Check sheet for the modelled part. Datum: model origin and axes. Units: mm. Face numbers are marked on the shaded views. A direction names the side the tool comes from. Round coordinates to 2 decimals unless told otherwise and drop trailing zeros. Write each loop counter-clockwise with the first axis right and the second up, starting at its lowest first coordinate (ties: lowest second). Pieces come first, ordered by that corner, then holes. Notation, with made-up numbers: (9, 67) -> (13, 67) arc R7 cw to (13, 80) -> close; hole circle Ø7 at (54, 64.25). An arc over 180 degrees is marked (long way). Answer as a JSON object with one key per item and string values. Group by question number.
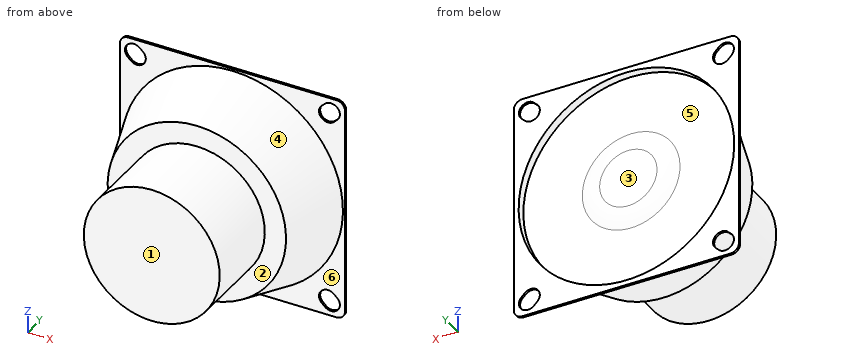
```python
from build123d import *

# Parameters (mm, degrees)
ESQUISSE2_R             = 16
BOSS_EXTRU_1_DEPTH      = 19
ESQUISSE3_R             = 21
BOSS_EXTRU_2_DEPTH      = 15
D_POUILLE1_ANGLE        = 18.5
BOSS_EXTRU_3_DEPTH      = 0.5
ESQUISSE5_R             = 25.375
ENL_V_MAT_EXTRU_1_DEPTH = 2
ESQUISSE6_R             = 11.5
BOSS_EXTRU_4_DEPTH      = 1.2
CONG_1_R                = 10
ENL_V_MAT_EXTRU_2_DEPTH = 10


with BuildPart() as part:
    # Esquisse2 → Boss.-Extru.1 (new body)
    with BuildSketch(Plane(origin=(0, 0, 0), x_dir=(1, 0, 0), z_dir=(0, 1, 0))):
        with Locations(Location((0, 0, 0), (0, 0, 270))):
            Circle(ESQUISSE2_R)
    extrude(amount=BOSS_EXTRU_1_DEPTH)

    # Esquisse3 → Boss.-Extru.2 (add)
    with BuildSketch(Plane(origin=(0, 19, 0), x_dir=(1, 0, 0), z_dir=(0, 1, 0))):
        with Locations(Location((0, 0, 0), (0, 0, 270))):
            Circle(ESQUISSE3_R)
    extrude(amount=BOSS_EXTRU_2_DEPTH)

    # Dépouille1
    d_pouille1_faces = [part.faces().sort_by_distance(p)[0] for p in [
        (0, 26.5, -21),
    ]]
    draft(d_pouille1_faces, Plane(origin=(0, 19, 0), x_dir=(0, 0, -1), z_dir=(0, -1, 0)), D_POUILLE1_ANGLE)

    # Esquisse4 → Boss.-Extru.3 (add)
    with BuildSketch(Plane(origin=(0, 34, 0), x_dir=(1, 0, 0), z_dir=(0, 1, 0))):
        with BuildLine():
            Line((-24.5, 26.5), (24.5, 26.5))
            ThreePointArc((24.5, 26.5), (25.914213562, 25.914213562), (26.5, 24.5))
            Line((26.5, 24.5), (26.5, -24.5))
            ThreePointArc((26.5, -24.5), (25.914213562, -25.914213562), (24.5, -26.5))
            Line((24.5, -26.5), (-24.5, -26.5))
            ThreePointArc((-24.5, -26.5), (-25.914213562, -25.914213562), (-26.5, -24.5))
            Line((-26.5, -24.5), (-26.5, 24.5))
            ThreePointArc((-26.5, 24.5), (-25.914213562, 25.914213562), (-24.5, 26.5))
        make_face()
    extrude(amount=BOSS_EXTRU_3_DEPTH)

    # Esquisse5 → Enlèv. mat.-Extru.1 (cut)
    with BuildSketch(Plane(origin=(0, 34.5, 0), x_dir=(1, 0, 0), z_dir=(0, 1, 0))):
        with Locations(Location((0, 0, 0), (0, 0, 270))):
            Circle(ESQUISSE5_R)
    extrude(amount=-ENL_V_MAT_EXTRU_1_DEPTH, mode=Mode.SUBTRACT)

    # Esquisse6 → Boss.-Extru.4 (add)
    with BuildSketch(Plane(origin=(0, 32.5, 0), x_dir=(1, 0, 0), z_dir=(0, 1, 0))):
        with Locations(Location((0, 0, 0), (0, 0, 270))):
            Circle(ESQUISSE6_R)
    extrude(amount=BOSS_EXTRU_4_DEPTH)

    # Congé1
    # the kernel refuses this fillet: 10 mm, written as the material it takes off along each edge
    with BuildSketch(Plane(origin=(0, 33.7, 0), x_dir=(0, 0, 1), z_dir=(-1, 0, 0))) as cong_1_piece_1:
        with BuildLine():
            CenterArc((6.750263165, -10), CONG_1_R, 61.642363424, 28.357636576)
            Line((6.750263165, 0), (6.750263165, 0.2))
            Line((6.750263165, 0.2), (11.5, 0.2))
            Line((11.5, 0.2), (11.7, 0))
            ThreePointArc((11.7, 0), (11.7, -0.6), (11.594994737, -1.024))
            Line((11.594994737, -1.024), (11.5, -1.2))
        make_face()
    revolve(axis=Axis((0, 33.7, 0), (0, 1, 0)), mode=Mode.SUBTRACT)

    # Esquisse7 → Enlèv. mat.-Extru.2 (cut)
    with BuildSketch(Plane(origin=(0, 34.5, 0), x_dir=(1, 0, 0), z_dir=(0, 1, 0))):
        with BuildLine():
            Line((21.024040871, 24.065615546), (21.74268552, 24.760993047))
            ThreePointArc((21.74268552, 24.760993047), (24.712132034, 24.712132034), (24.663271022, 21.74268552))
            Line((24.663271022, 21.74268552), (23.944626373, 21.04730802))
            ThreePointArc((23.944626373, 21.04730802), (20.975179858, 21.096169032), (21.024040871, 24.065615546))
        make_face()
        with BuildLine():
            Line((-21.024040871, 24.065615546), (-21.74268552, 24.760993047))
            ThreePointArc((-21.74268552, 24.760993047), (-24.712132034, 24.712132034), (-24.663271022, 21.74268552))
            Line((-24.663271022, 21.74268552), (-23.944626373, 21.04730802))
            ThreePointArc((-23.944626373, 21.04730802), (-20.975179858, 21.096169032), (-21.024040871, 24.065615546))
        make_face()
        with BuildLine():
            Line((21.024040871, -24.065615546), (21.74268552, -24.760993047))
            ThreePointArc((21.74268552, -24.760993047), (24.712132034, -24.712132034), (24.663271022, -21.74268552))
            Line((24.663271022, -21.74268552), (23.944626373, -21.04730802))
            ThreePointArc((23.944626373, -21.04730802), (20.975179858, -21.096169032), (21.024040871, -24.065615546))
        make_face()
        with BuildLine():
            Line((-21.024040871, -24.065615546), (-21.74268552, -24.760993047))
            ThreePointArc((-21.74268552, -24.760993047), (-24.712132034, -24.712132034), (-24.663271022, -21.74268552))
            Line((-24.663271022, -21.74268552), (-23.944626373, -21.04730802))
            ThreePointArc((-23.944626373, -21.04730802), (-20.975179858, -21.096169032), (-21.024040871, -24.065615546))
        make_face()
    extrude(amount=-ENL_V_MAT_EXTRU_2_DEPTH, mode=Mode.SUBTRACT)


solid = part.part
```
(1) Section check C-C on y = 27.5. Record the cut outline in (x, z).
(2) Section check B-B on x = 23. State how many separate pieces and enclosed holes the cut face has, then the cut area to 3 significant figures.
(3) Release check for a two-part mould opening along Z. For the marked faces 4, 5 and 6 record: pulls with the +Z half, pulls with the -Z half, needs draft (parallel to the pull), parting line crosses it, or undercut.
(4) Go/stop test with flat-tipped pins: pin 1 Ø8 at (x, y) = (19, 17.5) entering from +Z; pin 2 Ø7 at (x, z) = (-2, 3) entering from +Y; pin 3 Ø1 at (x, y) = (-0.5, 29.5) entering from -Z. Record where each tip stops, or that it passes through.
(5) Access from +Z, -Z, +X, -X, +Y, -Y to the whole of each face (thin tool, end or side, straight path). Record for the marked faces 1, 2 and 3.
(6) Section check A-A on y = 8.5. Record the cut outline in (x, z).
(7) Scan lines: line 1 along Y through (x, z) = (-23, -13); line 2 along Y through (x, z) = (11.5, -8); line 3 along Z through (x, y) = (0.5, 4.5). Record each from-to range of solid material in increasing order.
Data:
{
 "1": {"outline": "circle Ø47.69 at (0, 0)"},
 "2": {"separate pieces": "3", "enclosed holes": "0", "area": "123 mm²"},
 "3": {"face 4": "parting line crosses it", "face 5": "undercut", "face 6": "needs draft"},
 "4": {"pin 1": "stops at z = 14.4", "pin 2": "stops at y = 33.7", "pin 3": "stops at z = -24.68"},
 "5": {"face 1": "+Z, -Z, +X, -X, -Y", "face 2": "-Y", "face 3": "+Y"},
 "6": {"outline": "circle Ø32 at (0, 0)"},
 "7": {"line 1": "y = 34 to 34.5", "line 2": "y = 0 to 32.5", "line 3": "z = -15.99 to 15.99"}
}
